Autodesk Inventor part; units mm, degrees
ref_plane "YZ Plane" through (0, 0, 0) normal (1, 0, 0) x (0, 1, 0)
ref_plane "XZ Plane" through (0, 0, 0) normal (0, 1, 0) x (-1, 0, 0)
ref_plane "XY Plane" through (0, 0, 0) normal (0, 0, 1) x (1, 0, 0)
sketch "Sketch1" plane through (0, 0, 0) normal (0, 1, 0) x (-1, 0, 0)
  circle A0 centre (0, 0) radius 66.5
  dimension "d0" = 133
extrude "Extrusion1" add sketch "Sketch1" along normal blind 3
sketch "Sketch2" plane through (0, 3, 0) normal (0, 1, 0) x (1, 0, 0)
  circle A0 centre (0, 0) radius 55
  circle A1 centre (-60, 0) radius 1.5
  circle A2 centre (-30, -51.9615) radius 1.5
  circle A3 centre (30, -51.9615) radius 1.5
  circle A4 centre (60, 0) radius 1.5
  circle A5 centre (30, 51.9615) radius 1.5
  circle A6 centre (-30, 51.9615) radius 1.5
  dimension "d3" = 110
  dimension "d4" = 3
  dimension "d5" = 60
  dimension "d8" = 360
extrude "Extrusion2" cut sketch "Sketch2" against normal blind 3 contours A1 | A2 | A3 | A4 | A5 | A6
fillet "Fillet1" radius 2 1 edges at (66.5, 3, 0)
properties part number "Top"
Geometry: final body of the model. Coordinates: model frame, mm. Give positions to 0.01 mm unless a question says otherwise; leave off trailing zeros. Write each loop counter-clockwise with the first axis right and the second up, starting at its lowest first coordinate (ties: lowest second). Pieces come first, ordered by that corner, then holes.
(1) Ray query, line 1 (Z direction, x = 30, y = 0.9); line 2 (Z direction, x = 30, y = 1.95); line 3 (Y direction, x = 48.5, z = 43). Return the intervals inside material, ascending.
(2) First-contact query: P1, Ø1, axis at x = 51.5, y = 2, coming from the +Z side; P2, Ø1, axis at x = 33, y = 0.5, coming from the +Z side. Flat tips, straight axial feed; report the tip coordinate or a pass-through.
(3) Mould query, pull axis X, two halves, no side actions, for faces 1 (the cylindrical face through (-35.75, 0.493, -56.073)), 2 (the cylindrical face through (-58.57, 1.52, -0.45)), 3 (the flat face through (1, 3, 1)). Classes: released by +X, released by -X, zero draft, split by the parting line, or undercut.
(4) Cut plane A-A, the plane y = 2. Return loops of the section in (x, z).
Values follow:
1. line 1: z = -59.35 to -53.46, -50.46 to 50.46, 53.46 to 59.35
1. line 2: z = -59.08 to -53.46, -50.46 to 50.46, 53.46 to 59.08
1. line 3: y = 0 to 2.97
2. P1: stops at z = 42.37
2. P2: stops at z = 58.02
3. face 1: split by the parting line
3. face 2: undercut
3. face 3: zero draft
4. outline: circle Ø132.46 at (0, 0); hole circle Ø3 at (-60, 0); hole circle Ø3 at (-30, -51.96); hole circle Ø3 at (-30, 51.96); hole circle Ø3 at (30, -51.96); hole circle Ø3 at (30, 51.96); hole circle Ø3 at (60, 0)
